```python
from build123d import *

# Parameters (mm, degrees)
SKETCH1_W           = 10
SKETCH1_H           = 10
BOSS_EXTRUDE1_DEPTH = 14
SKETCH2_R           = 5
BOSS_EXTRUDE2_DEPTH = 20


with BuildPart() as part:
    # Sketch1 → Boss-Extrude1 (new body)
    with BuildSketch(Plane(origin=(0, 0, 0), x_dir=(1, 0, 0), z_dir=(0, 1, 0))):
        with Locations((5, -5)):
            Rectangle(SKETCH1_W, SKETCH1_H)
    boss_extrude1 = extrude(amount=BOSS_EXTRUDE1_DEPTH)

    # Sketch2 → Boss-Extrude2 (add)
    with BuildSketch(Plane.XY):
        with Locations((5, 14)):
            Circle(SKETCH2_R)
        with Locations((5, 0)):
            Circle(SKETCH2_R)
    boss_extrude2 = extrude(amount=BOSS_EXTRUDE2_DEPTH)

    # Mirror1: Boss-Extrude1, Boss-Extrude2 across plane
    add(boss_extrude1.mirror(Plane(origin=(0, 14, 0), x_dir=(1, 0, 0), z_dir=(0, 0, 1))))
    add(boss_extrude2.mirror(Plane(origin=(0, 14, 0), x_dir=(1, 0, 0), z_dir=(0, 0, 1))))


solid = part.part
```
The listing builds one solid part. Answer for the finished solid, in the listing's coordinates (mm). A direction names the side the tool comes from. Coordinates: 2 decimals unless noted, no trailing zeros. Loops run counter-clockwise (first coordinate to the right, second up) from the corner with the lowest first, then second, coordinate; pieces in that order, holes last. Notation, with made-up numbers: (59, -22) - (110, -22) arc R21 cw to (110, -1) - close; hole circle Ø7 at (56, 0.5). An arc over 180 degrees is marked (long way). Use a Markdown table: item, result. Add a question column.
1) Find the intervals of material crossed by line 1 (X direction, y = 14.25, z = 16); line 2 (Y direction, x = 5.75, z = -14); line 3 (Y direction, x = 6.5, z = 15), in increasing order.
2) The mould has two halves that part along Y. Classify faces 1 (the flat face through (5, 7, -10)), 2 (the flat face through (10, 7, 0)): released by +Y, released by -Y, zero draft, split by the parting line, or undercut.
3) The part is cut by section B-B, the plane x = 5. Give the vertices of the cut face in (y, z), and give its area (3 significant figures).
4) The part is cut by section D-D, the plane z = -2. Give the vertices of the cut face in (x, y).
5) For faces 3 (the flat face through (5, 0, -20)), 4 (the flat face through (5, 7, 10)), determine the directions among +Z, -Z, +X, -X, +Y, -Y from which every point of the face is accessible in a straight line to the end or side of a thin tool.
6) Given pin 1 (3 mm diameter, centred on x = 7, z = -7, fed in from +Y); pin 2 (1 mm diameter, centred on x = 3, z = 13, fed in from -Y); pin 3 (5 mm diameter, centred on x = 8.5, z = 10, fed in from -Y), each flat-ended and moving along its own axis, determine where each tip first touches the part or whether it passes through.
7) The part is cut by section C-C, the plane y = 9.5. Give the vertices of the cut face in (x, z).
8) The part is cut by section A-A, the plane z = 14.5. Give the vertices of the cut face in (x, y), and give its area (3 significant figures).
Here are the results:
| question | item | result |
|---|---|---|
| 1 | line 1 | x = 0.01 to 9.99 |
| 1 | line 2 | y = -4.94 to 4.94, 9.06 to 18.94 |
| 1 | line 3 | y = -4.77 to 4.77, 9.23 to 18.77 |
| 2 | face 1 | undercut |
| 2 | face 2 | zero draft |
| 3 | outline | (-5, -20) - (5, -20) - (5, -10) - (9, -10) - (9, -20) - (19, -20) - (19, 20) - (9, 20) - (9, 10) - (5, 10) - (5, 20) - (-5, 20) - close |
| 3 | area | 880 mm^2 |
| 4 | outline | (0, 0) arc R5 ccw to (10, 0) - (10, 14) arc R5 ccw to (0, 14) - close |
| 5 | face 3 | -Z, +X, -X, +Y, -Y |
| 5 | face 4 | +Z |
| 6 | pin 1 | stops at y = 18.97 |
| 6 | pin 2 | stops at y = -4.77 |
| 6 | pin 3 | stops at y = -4.9 |
| 7 | outline | (0, -10) - (2.82, -10) - (2.82, -20) - (7.18, -20) - (7.18, -10) - (10, -10) - (10, 10) - (7.18, 10) - (7.18, 20) - (2.82, 20) - (2.82, 10) - (0, 10) - close |
| 8 | outline | circle Ø10 at (5, 0); circle Ø10 at (5, 14) |
| 8 | area | 157 mm^2 |
